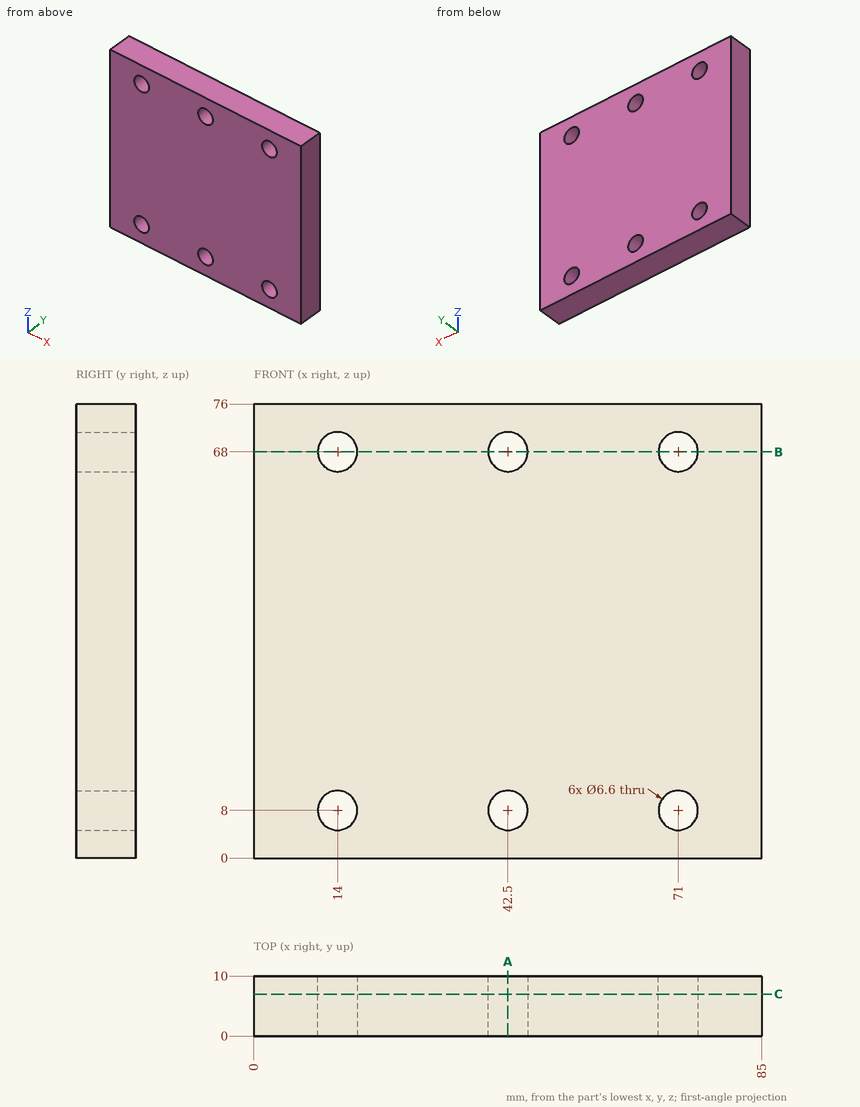
Here's the drawing with two shaded views (mm, measured from the low corner). I have some questions. Round coordinates to 2 decimals unless told otherwise and drop trailing zeros. Order: outer loops, then holes, each group sorted by start corner. A loop starts at its lowest first (then second) coordinate and runs counter-clockwise, first axis right, second up. Notation, with made-up numbers: M 10,64 L 39,64 A5 ccw 39,70 Z; hole C 77.25,43 d4. An arc over 180 degrees is marked long. Answer in a Markdown table with one row per item.
Item 1: Imagine slicing it at B-B, the plane z = 68. Write out the boundary of the cut face in (x, y).
A:
| item | result |
|---|---|
| outline | M 0,0 L 10.7,0 L 10.7,10 L 0,10 Z; M 17.3,0 L 39.2,0 L 39.2,10 L 17.3,10 Z; M 45.8,0 L 67.7,0 L 67.7,10 L 45.8,10 Z; M 74.3,0 L 85,0 L 85,10 L 74.3,10 Z |
Item 2: Imagine slicing it at C-C, the plane y = 7. Write out the boundary of the cut face in (x, z).
A:
| item | result |
|---|---|
| outline | M 0,0 L 85,0 L 85,76 L 0,76 Z; hole C 14,8 d6.6; hole C 14,68 d6.6; hole C 42.5,8 d6.6; hole C 42.5,68 d6.6; hole C 71,8 d6.6; hole C 71,68 d6.6 |
Item 3: I'm going to push a flat-ended pin straight in: pin 1 (5.5 mm diameter, centred on x = 71, z = 68, fed in from +Y). Where does the tip first touch, or does it pass through?
A:
| item | result |
|---|---|
| pin 1 | passes through |
Item 4: Imagine slicing it at A-A, the plane x = 42.5. Write out the boundary of the cut face in (y, z), and give its area (3 significant figures).
A:
| item | result |
|---|---|
| outline | M 0,0 L 10,0 L 10,4.7 L 0,4.7 Z; M 0,11.3 L 10,11.3 L 10,64.7 L 0,64.7 Z; M 0,71.3 L 10,71.3 L 10,76 L 0,76 Z |
| area | 628 mm2 |
Item 5: If I drill on L1, parallel to Z at x = 42.5, y = 6.25; L2, parallel to Z at x = 44, y = 3, over which ranges is the centre line in solid material (lowest first)? Write a range as from..to.
A:
| item | result |
|---|---|
| L1 | z = 0..4.7, 11.3..64.7, 71.3..76 |
| L2 | z = 0..5.06, 10.94..65.06, 70.94..76 |
